Check sheet for the modelled part. Datum: model origin and axes. Units: mm. A direction names the side the tool comes from. Give positions to 0.01 mm unless a question says otherwise; leave off trailing zeros. Order: outer loops, then holes, each group sorted by start corner. A loop starts at its lowest first (then second) coordinate and runs counter-clockwise, first axis right, second up.
from build123d import *

# Parameters (mm, degrees)
SKETCH1_R               = 35
BOSS_EXTRUDE1_DEPTH     = 10
SKETCH27_W              = 8.45046724
SKETCH27_H              = 8.572937779
CUT_EXTRUDE8_DEPTH      = 11
SKETCH34_R              = 2
CUT_EXTRUDE9_DEPTH      = 1
CUT_EXTRUDE9_DEPTH_BACK = 11
SKETCH35_R              = 2
CUT_EXTRUDE10_DEPTH     = 11
SKETCH36_R              = 2
CUT_EXTRUDE11_DEPTH     = 11
SKETCH37_R              = 2
CUT_EXTRUDE12_DEPTH     = 11
SKETCH39_R              = 32
CUT_EXTRUDE14_DEPTH     = 0.01


with BuildPart() as part:
    # Sketch1 → Boss-Extrude1 (new body)
    with BuildSketch(Plane(origin=(0, 0, 0), x_dir=(1, 0, 0), z_dir=(0, 1, 0))):
        Circle(SKETCH1_R)
    extrude(amount=BOSS_EXTRUDE1_DEPTH)

    # Sketch27 → Cut-Extrude8 (cut, through all)
    with BuildSketch(Plane(origin=(0, 10, 0), x_dir=(1, 0, 0), z_dir=(0, 1, 0))):
        with Locations((31.027560582, -0.794372815)):
            Rectangle(SKETCH27_W, SKETCH27_H)
    extrude(amount=-CUT_EXTRUDE8_DEPTH, mode=Mode.SUBTRACT)

    # Sketch34 → Cut-Extrude9 (cut, two sides)
    with BuildSketch(Plane(origin=(0, 10, 0), x_dir=(1, 0, 0), z_dir=(0, 1, 0))) as cut_extrude9_sk:
        with Locations((-17, 17)):
            Circle(SKETCH34_R)
    extrude(amount=CUT_EXTRUDE9_DEPTH, mode=Mode.SUBTRACT)
    extrude(cut_extrude9_sk.sketch, amount=-CUT_EXTRUDE9_DEPTH_BACK, mode=Mode.SUBTRACT)

    # Sketch35 → Cut-Extrude10 (cut, through all)
    with BuildSketch(Plane(origin=(0, 0, 0), x_dir=(-1, 0, 0), z_dir=(0, -1, 0))):
        with Locations((-17, 17)):
            Circle(SKETCH35_R)
    extrude(amount=-CUT_EXTRUDE10_DEPTH, mode=Mode.SUBTRACT)

    # Sketch36 → Cut-Extrude11 (cut, through all)
    with BuildSketch(Plane(origin=(0, 0, 0), x_dir=(-1, 0, 0), z_dir=(0, -1, 0))):
        with Locations((17, -17)):
            Circle(SKETCH36_R)
    extrude(amount=-CUT_EXTRUDE11_DEPTH, mode=Mode.SUBTRACT)

    # Sketch37 → Cut-Extrude12 (cut, through all)
    with BuildSketch(Plane.XZ):
        with Locations((17, 17)):
            Circle(SKETCH37_R)
    extrude(amount=-CUT_EXTRUDE12_DEPTH, mode=Mode.SUBTRACT)

    # Sketch39 → Cut-Extrude14 (cut)
    with BuildSketch(Plane(origin=(0, 10, 0), x_dir=(1, 0, 0), z_dir=(0, 1, 0))):
        Circle(SKETCH39_R)
    extrude(amount=-CUT_EXTRUDE14_DEPTH, mode=Mode.SUBTRACT)


solid = part.part
1) Section check A-A, the plane y = 2.75. Record the cut outline in (x, z).
Recorded:
outline: (26.8, -3.49) - (26.8, 5.08) - (34.63, 5.08) arc R35 ccw (long way) to (34.83, -3.49) - close; hole circle Ø4 at (-17, -17); hole circle Ø4 at (-17, 17); hole circle Ø4 at (17, -17); hole circle Ø4 at (17, 17)
2) Section check B-B, the plane x = -17. State how many separate pieces and enclosed holes the cut face has, then the cut area to 3 significant figures.
Recorded:
separate pieces: 3
enclosed holes: 0
area: 531 mm2
3) Draft check along X on faces 1 (the face through (31, 5, -3.492)), 2 (the face through (26.802, 5, 1)), 3 (the face through (-17, 5, 15)). Enter one of: +X half, -X half, draft (parallel to the pull), parting line (faces both ways), or undercut.
Recorded:
face 1: draft
face 2: +X half
face 3: undercut
4) Depth check by flat-ended pin: pin 1 Ø4 at (x, y) = (29, 6.5) entering from -Z; pin 2 Ø4 at (x, y) = (16, 8) entering from -Z; pin 3 Ø2 at (x, y) = (16, 4.5) entering from -Z; pin 4 Ø10 at (x, z) = (-2, 20.5) entering from -Y. Enter the tip coordinate at first touch or a pass-through.
Recorded:
pin 1: stops at z = -22.27
pin 2: stops at z = -32.08
pin 3: stops at z = -31.62
pin 4: stops at y = 0
5) Material ranges on L1, parallel to Z at x = 17, y = 0.75; L2, parallel to Y at x = -23.5, z = -2, recorded low to high.
Recorded:
L1: z = -30.59 to -19, -15 to 15, 19 to 30.59
L2: y = 0 to 9.99
6) Set-up check for faces 4 (the face through (-1, 0, 0)), 5 (the face through (31, 5, 5.081)): record each of +Z, -Z, +X, -X, +Y, -Y from which the full face is reachable in a straight line by a thin tool's end or side.
Recorded:
face 4: +Z, -Z, +X, -X, -Y
face 5: +X, +Y, -Y
